Work out the finished part from the listing and answer in its coordinate system (mm). A direction names the side the tool comes from. Round coordinates to 2 decimals unless told otherwise and drop trailing zeros. Order: outer loops, then holes, each group sorted by start corner. A loop starts at its lowest first (then second) coordinate and runs counter-clockwise, first axis right, second up. Notation, with made-up numbers: (72.5, -36.5) - (97.5, -36.5) arc R31 cw to (97.5, -3.5) - close; hole circle Ø1 at (62.25, -38). An arc over 180 degrees is marked (long way). Put each result on its own line as item: value.
Autodesk Inventor part; units mm, degrees
ref_plane "Work Plane6" through (14.4702, 32.0662, 39.5) normal (0, 0, 1) x (1, 0, 0)
ref_plane "Work Plane1" through (14.4702, 32.0662, 47.5) normal (0, 0, -1) x (-1, 0.0032, 0)
ref_plane "Work Plane2" through (14.4702, 32.0662, 46.35) normal (0, 0, -1) x (-1, 0.0032, 0)
ref_plane "Work Plane6" through (14.4702, 32.0662, 39.5) normal (0, 0, 1) x (1, 0, 0)
sketch "Sketch1" plane through (14.4702, 32.0662, 39.5) normal (0, 0, 1) x (1, 0, 0)
  point P0 (-14.4702, -32.0662)
ref_plane "Work Plane1" through (14.4702, 32.0662, 47.5) normal (0, 0, -1) x (-1, 0.0032, 0)
sketch "Sketch2" plane through (14.4702, 32.0662, 47.5) normal (0, 0, -1) x (-1, 0.0032, 0)
  line L0 (-3.06, 5.3) -> (3.06, 5.3)
  line L1 (3.06, 5.3) -> (6.1199, 0)
  line L2 (6.1199, 0) -> (3.06, -5.3)
  line L3 (3.06, -5.3) -> (-3.06, -5.3)
  line L4 (-3.06, -5.3) -> (-6.1199, 0)
  line L5 (-6.1199, 0) -> (-3.06, 5.3)
  circle A0 centre (0, 0) radius 8
  line L6 (-3.06, -5.3) -> (-3.06, 5.3)
  line L7 (-3.06, 5.3) -> (-8, 5.3)
  line L8 (-8, 5.3) -> (-8, -5.3)
  line L9 (-8, -5.3) -> (-3.06, -5.3)
  circle A1 centre (0, 0) radius 4.75
  point P0 (14.3663, -32.1129)
  point P1 (-5.9925, -5.3)
  point P2 (-5.9925, 5.3)
  point P3 (-3.06, 3.6331)
  point P4 (-3.06, -3.6331)
  point P5 (-3.06, -5.3)
  point P6 (-3.06, 5.3)
  point P7 (-3.06, -5.3)
  point P8 (-3.06, 5.3)
  point P9 (-3.06, -5.3)
  point P10 (-8, 0)
  point P11 (-3.06, 5.3)
  point P12 (-3.06, -5.3)
  dimension "d3" = 10.6
  dimension "d4" = 16
  dimension "d9" = 9.5
extrude "Extrusion1" add sketch "Sketch2" against normal blind 2.5 contours L7 A0 L9 L3 L2 L1 L0 | L6 A1 L4 L5 | L0 L1 L2 L3 L6 A1 | L5 L4 L9 A0 L7
ref_plane "Work Plane2" through (14.4702, 32.0662, 46.35) normal (0, 0, -1) x (-1, 0.0032, 0)
ref_plane "Work Plane4" through (20.4455, 26.7469, 47.5) normal (0.0032, 1, 0) x (1, -0.0032, 0)
sketch "Sketch5" plane through (20.4455, 26.7469, 47.5) normal (0.0032, 1, 0) x (1, -0.0032, 0)
  line L0 (-13.9925, -2.5) -> (2.0075, -2.5)
  line L1 (2.0075, 0) -> (-13.9925, 0)
  line L2 (-0.1528, -2.5) -> (-0.1528, 0)
  line L3 (-11.7789, -2.5) -> (-11.7789, 0)
  line L4 (2.0075, 0) -> (-13.9925, 0)
  point P0 (-20.3588, 47.5)
ref_plane "Work Plane7" through (-59.5298, 2.0662, -55) normal (0, 1, 0) x (1, 0, 0)
sketch "Sketch6" plane through (-59.5298, 2.0662, -55) normal (0, 1, 0) x (1, 0, 0)
  circle A0 centre (109, -95) radius 5.35
  circle A1 centre (109, -95) radius 5.75
  circle A2 centre (109, -95) radius 10.8507
  line L0 (109, -95) -> (98.8037, -91.2888)
  line L1 (109, -95) -> (119.1963, -91.2888)
  line L2 (109, -95) -> (98.1493, -95)
  line L3 (66.0434, -104.5) -> (82.0433, -104.5)
  line L4 (82.0433, -104.5) -> (114.2428, -104.5)
  line L5 (66, -105) -> (82, -105)
  line L6 (66, -104.5) -> (82, -104.5)
  line L7 (82, -105.5) -> (82.0433, -105.5)
  point P0 (59.5298, -55)
  point P1 (103.5968, -93.0334)
  point P2 (114.4032, -93.0334)
  point P3 (103.7572, -104.5)
  dimension "d12" = 11.5
  dimension "d13" = 20
  dimension "d14" = 160
extrude "Extrusion3" add sketch "Sketch6" along normal blind 2 contours L1 A2 L4 L2 A1 | L2 A2 L0 A1
ref_plane "Work Plane8" through (-59.5298, 2.0662, -55) normal (0, 1, 0) x (1, 0, 0)
sketch "Sketch7" plane through (-59.5298, 2.0662, -55) normal (0, 1, 0) x (1, 0, 0)
  line L0 (68.2541, -98.4179) -> (68.2541, -104.2594)
  line L1 (79.6782, -98.4179) -> (79.6782, -104.2594) construction
  line L2 (68.2541, -98.4179) -> (103.5968, -93.0334)
  line L3 (68.2541, -104.2594) -> (103.343, -104.2594)
  arc A0 (98.8037, -91.2888) -> (119.1963, -91.2888) centre (109, -95) ccw
  line L4 (103.5968, -93.0334) -> (98.8037, -91.2888)
  arc A1 (103.5968, -93.0334) -> (109, -100.75) centre (109, -95) ccw
  line L5 (103.343, -104.2594) -> (109, -100.75)
  arc A2 (98.21, -93.8541) -> (103.343, -104.2594) centre (109, -95) ccw
  line L6 (103.343, -104.2594) -> (114.657, -104.2594)
  circle A3 centre (109, -95) radius 10.8507
  point P0 (59.5298, -55)
loft "Loft1" add profiles "Sketch7", "Sketch5" contours L2 A0 L3 L0 / all
extrude "Extrusion4" add sketch "Sketch7" along normal blind 2 contours L2 A0 L3 L0
ref_plane "Work Plane5" through (-59.5298, 2.0662, -55) normal (0, 1, 0) x (1, 0, 0)
sketch "Sketch9" plane through (-59.5298, 2.0662, -55) normal (0, 1, 0) x (1, 0, 0)
  point P0 (59.5298, -55)
extrude "Extrusion6" cut sketch "Sketch7" along normal blind 10 contours L6 A0
properties part number "Pot_mount_best"
1) A cutting plane is placed at B-B on y = 35.5. Write down the section's boundary in (x, z), then the cut area to 3 significant figures.
Findings below:
outline: (7.24, 47.5) - (11.19, 47.5) - (11.19, 50) - (7.24, 50) - close; (17.75, 47.5) - (21.7, 47.5) - (21.7, 50) - (17.75, 50) - close
area: 19.7 mm2
2) A cutting plane is placed at A-A on y = 28.5. Write down the section's boundary in (x, z), then the cut area to 3 significant figures.
Findings below:
outline: (7.31, 47.5) - (11.33, 47.5) - (11.33, 50) - (7.31, 50) - close; (17.61, 47.5) - (21.63, 47.5) - (21.63, 50) - (17.61, 50) - close
area: 20.1 mm2
3) Straight lines are drawn through the part: L1, parallel to Y at x = 43, z = 43.75; L2, parallel to Z at x = 14, y = 27; L3, parallel to Z at x = 19, y = 11. For each, find the intervals that lie inside material, in ascending order. Write a range as from..to.
Findings below:
L1: y = 2.07..4.07
L2: z = 47.5..50
L3: z = 43.61..49.53
4) Given pin 1 Ø8 at (x, z) = (38.5, 43) entering from +Y; pin 2 Ø3 at (y, z) = (21, 42.5) entering from -X; pin 3 Ø5 at (x, y) = (25, 19.5) entering from -Z; pin 4 Ø8 at (x, z) = (46, 44.5) entering from -Y, each flat-ended and moving along its own axis, determine where each tip first touches the part or whether it passes through.
Findings below:
pin 1: stops at y = 7.8
pin 2: passes through
pin 3: stops at z = 44.29
pin 4: stops at y = 2.07
5) For faces 1 (the flat face through (57.24, 3.05, 37.17)), 2 (the cylindrical face through (9.944, 33.507, 48.732)), 3 (the flat face through (15, 38, 47.5)), determine the directions among +Z, -Z, +X, -X, +Y, -Y from which every point of the face is accessible in a straight line to the end or side of a thin tool.
Findings below:
face 1: -Z, +Y, -Y
face 2: +Z, -Z
face 3: -Z, +X, -X, +Y
6) For a pull along X with two mould halves and no side action, classify faces 4 (the cylindrical face through (49.62, 3.05, 45.75)), 5 (the cylindrical face through (38.895, 3.052, 37.571)), 6 (the cylindrical face through (15.5, 40, 48.7)), 7 (the flat face through (41.7, 3.05, 37.17)) as pulls with the +X half, pulls with the -X half, needs draft (parallel to the pull), parting line crosses it, or undercut.
Findings below:
face 4: undercut
face 5: pulls with the -X half
face 6: parting line crosses it
face 7: undercut
